Build history of the part. All positions in model axes, mm. A direction names the side the tool comes from. Coordinates: 2 decimals unless noted, no trailing zeros. Loops run counter-clockwise (first coordinate to the right, second up) from the corner with the lowest first, then second, coordinate; pieces in that order, holes last. Notation, with made-up numbers: (84, 40) - (120, 40) arc R22 cw to (120, 48) - close; hole circle Ø6 at (46.25, -7.5). An arc over 180 degrees is marked (long way). One line per item, written item: value.
```python
from build123d import *

# Parameters (mm, degrees)
F1_DEPTH  = 32
F2_R      = 5.5
F3_DEPTH  = 13.001
F4_R      = 5.5
F5_DEPTH  = 13.001
F6_R      = 6.5
F7_DEPTH  = 88.001
F9_DEPTH  = 13.001
F11_DEPTH = 13.001
F14_DEPTH = 63
F17_DEPTH = 63
F18_W     = 25
F18_H     = 4.4557750225
F19_DEPTH = 32.001


with BuildPart() as f1:
    # F0 (on Front) → F1 (new body)
    with BuildSketch(Plane.XZ):
        Polygon((0, 13), (0, 0), (39, 0), (39, 17), (74, 17), (74, 0), (113, 0), (113, 13), (88, 13), (88, 64), (69, 64), (69, 30), (44, 30), (44, 64), (25, 64), (25, 13), align=None)
    extrude(amount=F1_DEPTH)

    # F2 (on face) → F3 (cut, through all)
    with BuildSketch(Plane.XY.offset(13)):
        with Locations((100, -13)):
            Circle(F2_R)
    extrude(amount=-F3_DEPTH, mode=Mode.SUBTRACT)

    # F4 (on face) → F5 (cut, through all)
    with BuildSketch(Plane.XY.offset(13)):
        with Locations((13, -13)):
            Circle(F4_R)
    extrude(amount=-F5_DEPTH, mode=Mode.SUBTRACT)

    # F6 (on face) → F7 (cut, through all)
    with BuildSketch(Plane.YZ.offset(88)):
        with Locations((-16, 46)):
            Circle(F6_R)
    extrude(amount=-F7_DEPTH, mode=Mode.SUBTRACT)

    # F8 (on face) → F9 (cut, through all)
    with BuildSketch(Plane.XY.offset(13)):
        Polygon((103, -32), (113, -32), (113, -22), align=None)
    extrude(amount=-F9_DEPTH, mode=Mode.SUBTRACT)

    # F10 (on face) → F11 (cut, through all)
    with BuildSketch(Plane.XY.offset(13)):
        Polygon((10, -32), (0, -22), (0, -32), align=None)
    extrude(amount=-F11_DEPTH, mode=Mode.SUBTRACT)

    # F16 (on face) → F17 (join)
    with BuildSketch(Plane.YZ.offset(88)):
        with BuildLine():
            Line((-32, 64), (0, 64))
            ThreePointArc((0, 64), (-16, 67.8712351675), (-32, 64))
        make_face()
    extrude(amount=-F17_DEPTH)

    # F18 (on Front) → F19 (cut, through all)
    with BuildSketch(Plane.XZ):
        with Locations((56.5, 66.2278875113)):
            Rectangle(F18_W, F18_H)
    extrude(amount=F19_DEPTH, mode=Mode.SUBTRACT)


with BuildPart() as f14:
    # F13 (on face) → F14 (new body)
    with BuildSketch(Plane.YZ.offset(88)):
        with BuildLine():
            Line((-32, 64), (0, 64))
            ThreePointArc((0, 64), (-16, 67.8712351675), (-32, 64))
        make_face()
    extrude(amount=-F14_DEPTH)


solid = f1.part
```
Item 1: Drop flat-ended pins along their axis: P1, Ø3, axis at y = -26, z = 36.5, coming from the -X side; P2, Ø12.5, axis at x = 100, y = -13, coming from the +Z side; P3, Ø7.5, axis at x = 56, y = -19.5, coming from the +Z side. Give the stop position or say it passes through.
Check result:
P1: stops at x = 25
P2: stops at z = 13
P3: stops at z = 30
Item 2: Cut at B-B, the plane x = 100. Write the cut outline in (y, z).
Check result:
outline: (-32, 0) - (-18.5, 0) - (-18.5, 13) - (-32, 13) - close; (-7.5, 0) - (0, 0) - (0, 13) - (-7.5, 13) - close
Item 3: Pull direction X, two halves, no side cores. Call faces 1 (the face through (94.505, -12.758, 6.591)), 2 (the face through (56, 0, 25)), 3 (the face through (25, -16, 35)): released by +X, released by -X, zero draft, split by the parting line, or undercut.
Check result:
face 1: undercut
face 2: zero draft
face 3: released by -X
Item 4: Probe probe 1 along X at (y, z) = (-21, 41); probe 2 along Y at (x, z) = (100, 3); probe 3 along X at (y, z) = (-25, 20.5). List the from-to ranges inside material, lowest first. Write a range as from..to.
Check result:
probe 1: x = 25..44, 69..88
probe 2: y = -32..-18.5, -7.5..0
probe 3: x = 25..88
Item 5: Tool access for faces 4 (the face through (101, -19, 13)), 5 (the face through (44, -16, 53)), 6 (the face through (13, -19, 13)), 7 (the face through (39, -16, 8)): list every direction of +Z, -Z, +X, -X, +Y, -Y with a clear straight run to the whole face (end or side of a thin tool).
Check result:
face 4: +Z, +X, +Y, -Y
face 5: +Z, +Y, -Y
face 6: +Z, -X, +Y, -Y
face 7: -Z, +Y, -Y
Item 6: Cut at C-C, the plane z = 54. Write the cut outline in (x, y), then the cut area to 3 significant figures.
Check result:
outline: (25, -32) - (44, -32) - (44, 0) - (25, 0) - close; (69, -32) - (88, -32) - (88, 0) - (69, 0) - close
area: 1,220 mm^2
Item 7: Cut at D-D, the plane y = -13. Give the number of separate pieces and of enclosed holes in the cut face, then the cut area to 3 significant figures.
Check result:
separate pieces: 5
enclosed holes: 0
area: 2,650 mm^2
Item 8: Cut at A-A, the plane z = 10.5. Write the cut outline in (x, y).
Check result:
outline: (0, -22) - (10, -32) - (39, -32) - (39, 0) - (0, 0) - close; (74, -32) - (103, -32) - (113, -22) - (113, 0) - (74, 0) - close; hole circle Ø11 at (13, -13); hole circle Ø11 at (100, -13)
